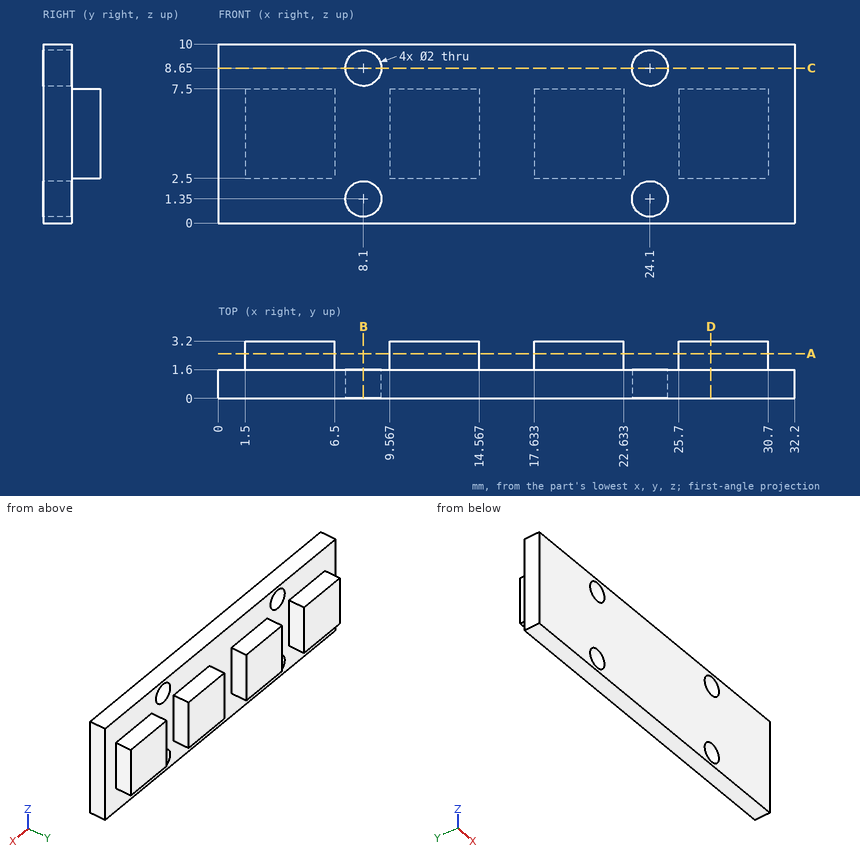
Here's the drawing with two shaded views (mm, measured from the low corner). I have some questions. Give positions to 0.01 mm unless a question says otherwise; leave off trailing zeros. Write each loop counter-clockwise with the first axis right and the second up, starting at its lowest first coordinate (ties: lowest second). Pieces come first, ordered by that corner, then holes. Notation, with made-up numbers: (18.25, 36.25) -> (64.25, 36.25) arc R25 ccw to (64.25, 49.25) -> close; hole circle Ø1 at (26.25, 40). An arc over 180 degrees is marked (long way). Answer as a JSON object with one key per item and string values. Group by question number.
Item 1: Suppose I cut it at A-A (y = 2.5). Please give me the cut outline in (x, z), plus the area to 3 significant figures.
Item 2: Suppose I cut it at C-C (z = 8.65). Please give me the cut outline in (x, y).
Item 3: I'm going to push flat-ended pins straight in: P1, Ø3, axis at x = 8.5, z = 8.5, coming from the +Y side; P2, Ø1.3, axis at y = 2.5, z = 4, coming from the +X side; P3, Ø0.8, axis at x = 29, y = 2.5, coming from the -Z side; P4, Ø2.5, axis at x = 8.1, z = 8.65, coming from the +Y side. Where does each tip first touch, or does it pass through?
Item 4: Please list where these lines run through material, in increasing order: line 1 (X direction, y = 2.5, z = 3); line 2 (X direction, y = 0.45, z = 8.65); line 3 (Z direction, x = 8, y = 1.5) (1 decimal). Write a range as [from, to].
Item 5: Suppose I cut it at B-B (x = 8.1). Please give me the cut outline in (y, z).
Item 6: Suppose I cut it at D-D (x = 27.5). Please give me the cut outline in (y, z).
Findings:
{
 "1": {"outline": "(1.5, 2.5) -> (6.5, 2.5) -> (6.5, 7.5) -> (1.5, 7.5) -> close; (9.57, 2.5) -> (14.57, 2.5) -> (14.57, 7.5) -> (9.57, 7.5) -> close; (17.63, 2.5) -> (22.63, 2.5) -> (22.63, 7.5) -> (17.63, 7.5) -> close; (25.7, 2.5) -> (30.7, 2.5) -> (30.7, 7.5) -> (25.7, 7.5) -> close", "area": "100 mm²"},
 "2": {"outline": "(0, 0) -> (7.1, 0) -> (7.1, 1.6) -> (0, 1.6) -> close; (9.1, 0) -> (23.1, 0) -> (23.1, 1.6) -> (9.1, 1.6) -> close; (25.1, 0) -> (32.2, 0) -> (32.2, 1.6) -> (25.1, 1.6) -> close"},
 "3": {"P1": "stops at y = 3.2", "P2": "stops at x = 30.7", "P3": "stops at z = 2.5", "P4": "stops at y = 1.6"},
 "4": {"line 1": "x = [1.5, 6.5], [9.57, 14.57], [17.63, 22.63], [25.7, 30.7]", "line 2": "x = [0, 7.1], [9.1, 23.1], [25.1, 32.2]", "line 3": "z = [0, 0.4], [2.3, 7.7], [9.6, 10]"},
 "5": {"outline": "(0, 0) -> (1.6, 0) -> (1.6, 0.35) -> (0, 0.35) -> close; (0, 2.35) -> (1.6, 2.35) -> (1.6, 7.65) -> (0, 7.65) -> close; (0, 9.65) -> (1.6, 9.65) -> (1.6, 10) -> (0, 10) -> close"},
 "6": {"outline": "(0, 0) -> (1.6, 0) -> (1.6, 2.5) -> (3.2, 2.5) -> (3.2, 7.5) -> (1.6, 7.5) -> (1.6, 10) -> (0, 10) -> close"}
}
